Answer from the drawing. Dimensions are ordinates in mm from the lowest x, y and z of the part. A direction names the side the tool comes from. Give positions to 0.01 mm unless a question says otherwise; leave off trailing zeros. Order: outer loops, then holes, each group sorted by start corner. A loop starts at its lowest first (then second) coordinate and runs counter-clockwise, first axis right, second up. Notation, with made-up numbers: (-34, 13) - (-14, 13) arc R20 ccw to (-14, 52) - close; hole circle Ø8 at (-37, -4.75). An arc over 180 degrees is marked (long way). Use a Markdown table: item, result. Add a question column.
1) The mould has two halves that part along X. Classify the marked faces 3, 4 and 5: released by +X, released by -X, zero draft, split by the parting line, or undercut.
2) Find section A-A, the plane y = 35. Determine the outline of the cut face in (x, z).
3) For the marked faces 1 and 2, determine the directions among +Z, -Z, +X, -X, +Y, -Y from which every point of the face is accessible in a straight line to the end or side of a thin tool.
4) Find section D-D, the plane x = 4.5. Determine the outline of the cut face in (y, z), plus the area to 3 significant figures.
5) Find section B-B, the plane x = 7.5. Determine the outline of the cut face in (y, z).
6) Find section C-C, the plane z = 3. Determine the outline of the cut face in (x, y), plus the area to 3 significant figures.
7) Straight lines are drawn through the part: line 1 (Y direction, x = 7.5, z = 9.65); line 2 (Y direction, x = 14.75, z = 5); line 3 (Z direction, x = 9.5, y = 28). For each, find the intervals that lie inside material, in ascending order.
8) A flat-ended cylindrical pin translates along its axis: pin 1 (2.5 mm diameter, centred on y = 25, z = 5, fed in from +X). Find the tip coordinate at first contact, or state that the pin passes through.
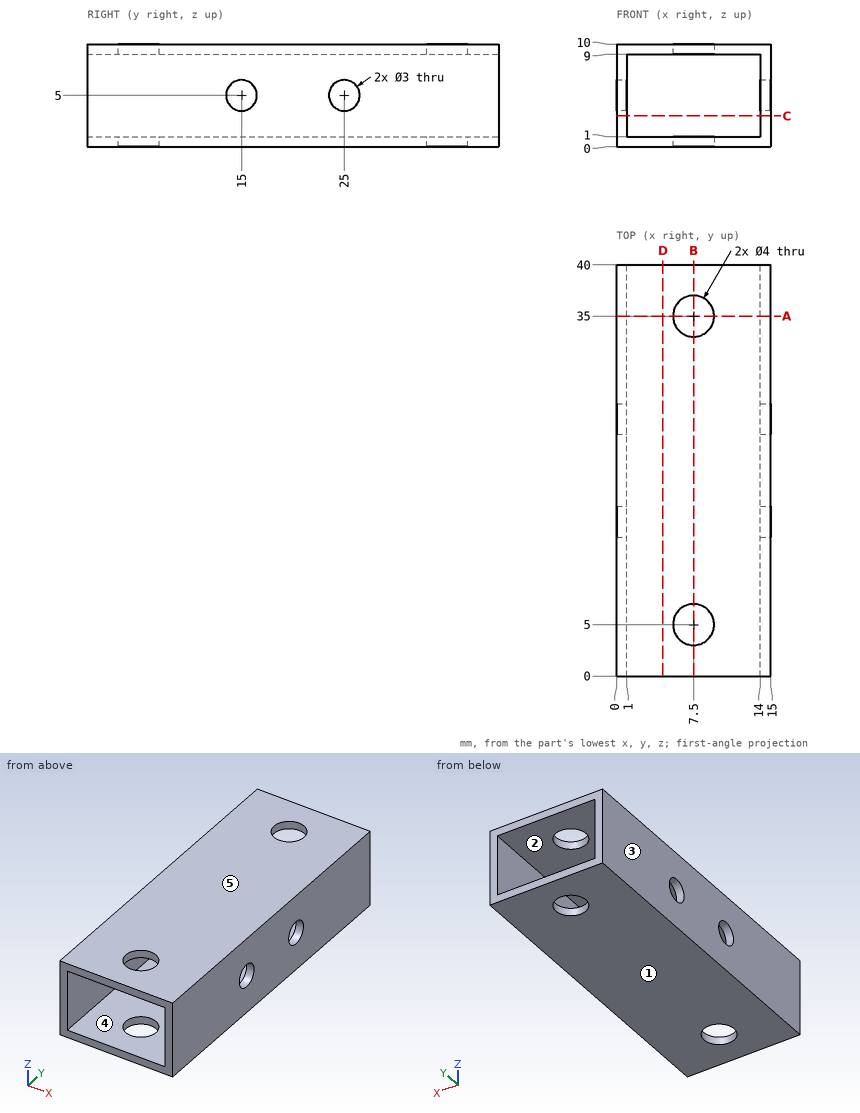
The answers:
| question | item | result |
|---|---|---|
| 1 | face 3 | released by -X |
| 1 | face 4 | undercut |
| 1 | face 5 | zero draft |
| 2 | outline | (0, 0) - (5.5, 0) - (5.5, 1) - (1, 1) - (1, 9) - (5.5, 9) - (5.5, 10) - (0, 10) - close; (9.5, 0) - (15, 0) - (15, 10) - (9.5, 10) - (9.5, 9) - (14, 9) - (14, 1) - (9.5, 1) - close |
| 3 | face 1 | -Z, +X, -X, +Y, -Y |
| 3 | face 2 | +Y, -Y |
| 4 | outline | (0, 0) - (40, 0) - (40, 1) - (0, 1) - close; (0, 9) - (40, 9) - (40, 10) - (0, 10) - close |
| 4 | area | 80.0 mm2 |
| 5 | outline | (0, 0) - (3, 0) - (3, 1) - (0, 1) - close; (0, 9) - (3, 9) - (3, 10) - (0, 10) - close; (7, 0) - (33, 0) - (33, 1) - (7, 1) - close; (7, 9) - (33, 9) - (33, 10) - (7, 10) - close; (37, 0) - (40, 0) - (40, 1) - (37, 1) - close; (37, 9) - (40, 9) - (40, 10) - (37, 10) - close |
| 6 | outline | (0, 0) - (1, 0) - (1, 40) - (0, 40) - close; (14, 0) - (15, 0) - (15, 40) - (14, 40) - close |
| 6 | area | 80.0 mm2 |
| 7 | line 1 | 0 to 3, 7 to 33, 37 to 40 |
| 7 | line 2 | 0 to 13.5, 16.5 to 23.5, 26.5 to 40 |
| 7 | line 3 | 0 to 1, 9 to 10 |
| 8 | pin 1 | through |
